Source: CAD feature listing. Evaluate the final solid. Frame: model axes, mm. Face numbers are marked on the shaded views. A direction names the side the tool comes from. Coordinates: 2 decimals unless noted, no trailing zeros. Order: outer loops, then holes, each group sorted by start corner. A loop starts at its lowest first (then second) coordinate and runs counter-clockwise, first axis right, second up.
Item 1: Ray query, line 1 (X direction, y = 0.2, z = 0); line 2 (X direction, y = 11.25, z = -23); line 3 (Y direction, x = -38.5, z = -34). Return the intervals inside material, ascending.
Item 2: Mould query, pull axis Z, two halves, no side actions, for the marked faces 3, 4 and 5. Classes: released by +Z, released by -Z, zero draft, split by the parting line, or undercut.
Item 3: Contact query for flat-ended pins moving along their axis: P1, Ø4, axis at x = 55, z = 18, coming from the +Y side; P2, Ø1.8, axis at x = 57, y = -1, coming from the -Z side; P3, Ø2, axis at y = 6, z = 22, coming from the +X side; P4, Ø2.5, axis at x = 55, y = 12.5, coming from the -Z side. Output: stop coordinate, or through.
Item 4: Reachability of the marked faces 1 and 2 from +Z, -Z, +X, -X, +Y, -Y: full face, straight path, thin tool, end or side. Return the list, or none.
Item 5: Section A-A on z = 0. Return the cut outline in (x, y), then the cut area to 3 significant figures.
Item 6: Section D-D on z = -14. Return the cut outline in (x, y).
Item 7: Section C-C on y = 16.75. Return the cut outline in (x, z).
Item 8: Section B-B on x = 24. Return the cut outline in (y, z).
from build123d import *

# Parameters (mm, degrees)
SKETCH1_W           = 99
SKETCH1_H           = 67
BOSS_EXTRUDE1_DEPTH = 23
SKETCH2_W           = 116
SKETCH2_H           = 69.2
BOSS_EXTRUDE2_DEPTH = 3.5
SKETCH3_W           = 116
SKETCH3_H           = 2.2
BOSS_EXTRUDE3_DEPTH = 23
SKETCH4_W           = 91
SKETCH4_H           = 11.969413233
BOSS_EXTRUDE4_DEPTH = 9.5
FILLET1_R           = 3
FILLET2_R           = 3
CUT_EXTRUDE1_DEPTH  = 9.5
CUT_EXTRUDE2_DEPTH  = 9.5
BOSS_EXTRUDE5_DEPTH = 2
SKETCH9_R           = 1.727966507
CUT_EXTRUDE3_DEPTH  = 76.193084788


with BuildPart() as part:
    # Sketch1 → Boss-Extrude1 (new body)
    with BuildSketch(Plane(origin=(0, 0, 0), x_dir=(1, 0, 0), z_dir=(0, 1, 0))):
        Rectangle(SKETCH1_W, SKETCH1_H)
    extrude(amount=BOSS_EXTRUDE1_DEPTH)

    # Sketch2 → Boss-Extrude2 (add)
    with BuildSketch(Plane.XZ):
        with Locations((0, 1.1)):
            Rectangle(SKETCH2_W, SKETCH2_H)
    extrude(amount=BOSS_EXTRUDE2_DEPTH)

    # Sketch3 → Boss-Extrude3 (add)
    with BuildSketch(Plane(origin=(0, 0, 0), x_dir=(1, 0, 0), z_dir=(0, 1, 0))):
        with Locations((0, -34.6)):
            Rectangle(SKETCH3_W, SKETCH3_H)
    extrude(amount=BOSS_EXTRUDE3_DEPTH)

    # Sketch4 → Boss-Extrude4 (add)
    with BuildSketch(Plane(origin=(0, 0, -33.5), x_dir=(-1, 0, 0), z_dir=(0, 0, -1))):
        with Locations((0, 5.984706617)):
            Rectangle(SKETCH4_W, SKETCH4_H)
    extrude(amount=BOSS_EXTRUDE4_DEPTH)

    # Fillet1
    fillet1_edges = [part.edges().sort_by_distance(p)[0] for p in [
        (0, 11.969413233, -43),
    ]]
    fillet(fillet1_edges, radius=FILLET1_R)

    # Fillet2
    fillet2_edges = [part.edges().sort_by_distance(p)[0] for p in [
        (58, 23, 34.6),
        (-58, 23, 34.6),
    ]]
    fillet(fillet2_edges, radius=FILLET2_R)

    # Sketch5 → Cut-Extrude1 (cut)
    with BuildSketch(Plane.XY.offset(35.7)):
        with BuildLine():
            Line((-54.5, 14), (-58, 14))
            Line((-58, 14), (-58, 9))
            Line((-58, 9), (-54.5, 9))
            ThreePointArc((-54.5, 9), (-52, 11.5), (-54.5, 14))
        make_face()
        with BuildLine():
            Line((58, 9), (54.5, 9))
            ThreePointArc((54.5, 9), (52, 11.5), (54.5, 14))
            Line((54.5, 14), (58, 14))
            Line((58, 14), (58, 9))
        make_face()
    extrude(amount=-CUT_EXTRUDE1_DEPTH, mode=Mode.SUBTRACT)

    # Sketch6 → Cut-Extrude2 (cut)
    with BuildSketch(Plane(origin=(0, 0, 0), x_dir=(1, 0, 0), z_dir=(0, 1, 0))):
        with BuildLine():
            Line((54.5, 16.5), (58, 16.5))
            Line((58, 16.5), (58, 11.5))
            Line((58, 11.5), (54.5, 11.5))
            ThreePointArc((54.5, 11.5), (52, 14), (54.5, 16.5))
        make_face()
        with BuildLine():
            Line((54.5, -11.5), (58, -11.5))
            Line((58, -11.5), (58, -16.5))
            Line((58, -16.5), (54.5, -16.5))
            ThreePointArc((54.5, -16.5), (52, -14), (54.5, -11.5))
        make_face()
        with BuildLine():
            Line((-58, -16.5), (-54.5, -16.5))
            ThreePointArc((-54.5, -16.5), (-52, -14), (-54.5, -11.5))
            Line((-54.5, -11.5), (-58, -11.5))
            Line((-58, -11.5), (-58, -16.5))
        make_face()
        with BuildLine():
            Line((-58, 11.5), (-54.5, 11.5))
            ThreePointArc((-54.5, 11.5), (-52, 14), (-54.5, 16.5))
            Line((-54.5, 16.5), (-58, 16.5))
            Line((-58, 16.5), (-58, 11.5))
        make_face()
    extrude(amount=-CUT_EXTRUDE2_DEPTH, mode=Mode.SUBTRACT)

    # Sketch8 → Boss-Extrude5 (add)
    with BuildSketch(Plane(origin=(0, 0, 0), x_dir=(1, 0, 0), z_dir=(0, 1, 0))):
        with BuildLine():
            Line((-57, -7), (-49.5, -7))
            Line((-49.5, -7), (-49.5, 7))
            Line((-49.5, 7), (-57, 7))
            ThreePointArc((-57, 7), (-57.707106781, 6.707106781), (-58, 6))
            Line((-58, 6), (-58, -6))
            ThreePointArc((-58, -6), (-57.707106781, -6.707106781), (-57, -7))
        make_face()
        with BuildLine():
            Line((49.5, -7), (49.5, 7))
            Line((49.5, 7), (57, 7))
            ThreePointArc((57, 7), (57.707106781, 6.707106781), (58, 6))
            Line((58, 6), (58, -6))
            ThreePointArc((58, -6), (57.707106781, -6.707106781), (57, -7))
            Line((57, -7), (49.5, -7))
        make_face()
    extrude(amount=BOSS_EXTRUDE5_DEPTH)

    # Sketch9 → Cut-Extrude3 (cut, through all)
    with BuildSketch(Plane(origin=(0, 2, 0), x_dir=(1, 0, 0), z_dir=(0, 1, 0))):
        with Locations(Location((-54.678466494, 0, 0), (0, 0, 270))):
            Circle(SKETCH9_R)
        with Locations(Location((54.678466494, 0, 0), (0, 0, 90))):
            Circle(SKETCH9_R)
    extrude(amount=-CUT_EXTRUDE3_DEPTH, mode=Mode.SUBTRACT)


solid = part.part
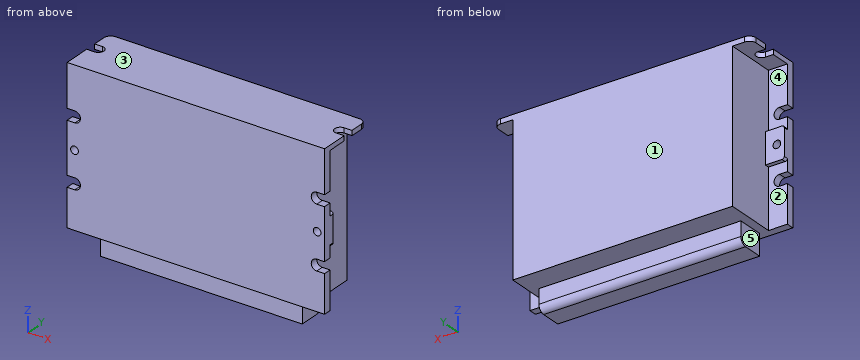
Answer list:
1. line 1: x = -58 to -56.41, -52.95 to 52.95, 56.41 to 58
1. line 2: x = -49.5 to 49.5
1. line 3: y = 0 to 11.97
2. face 3: released by +Z
2. face 4: undercut
2. face 5: zero draft
3. P1: stops at y = 0
3. P2: stops at z = -33.5
3. P3: stops at x = 49.5
3. P4: passes through
4. face 1: +Z, -Z, +X, -X, +Y
4. face 2: -Z, -X, +Y
5. outline: (-58, -3.5) - (-56.41, -3.5) - (-56.41, 2) - (-58, 2) - close; (-52.95, -3.5) - (52.95, -3.5) - (52.95, 2) - (49.5, 2) - (49.5, 23) - (-49.5, 23) - (-49.5, 2) - (-52.95, 2) - close; (56.41, -3.5) - (58, -3.5) - (58, 2) - (56.41, 2) - close
5. area: 2,680 mm2
6. outline: (-52, -3.5) - (52, -3.5) - (52, 0) - (49.5, 0) - (49.5, 23) - (-49.5, 23) - (-49.5, 0) - (-52, 0) - close
7. outline: (-58, 33.5) - (-49.5, 33.5) - (-49.5, -33.5) - (49.5, -33.5) - (49.5, 33.5) - (58, 33.5) - (58, 35.7) - (-58, 35.7) - close
8. outline: (-3.5, -33.5) - (0, -33.5) - (0, -43) - (8.97, -43) arc R3 ccw to (11.97, -40) - (11.97, -33.5) - (23, -33.5) - (23, 35.7) - (-3.5, 35.7) - close
